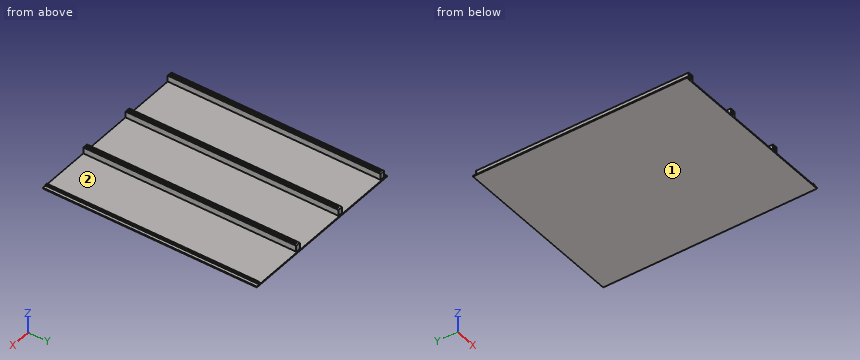
from build123d import *

# Parameters (mm, degrees)
F0_W     = 5.2
F0_H     = 226.71
F1_DEPTH = 2
F3_DEPTH = 4.5
F4_W     = 1.2
F4_H     = 2.1
F5_DEPTH = 25
F6_W     = 185.5
F6_H     = 227.71
F6_W_2   = 2.7
F7_DEPTH = 1
F8_W     = 2
F8_H     = 226.618603
F9_DEPTH = 1
F10_SIZE = 1


with BuildPart() as f1:
    # F0 (on Top) → F1 (new body)
    with BuildSketch(Plane.XY):
        with Locations((2.6, 113.355)):
            Rectangle(F0_W, F0_H)
        with Locations((63.6, 113.355)):
            Rectangle(F0_W, F0_H)
        with Locations((124.6, 113.355)):
            Rectangle(F0_W, F0_H)
    extrude(amount=F1_DEPTH)

    # F2 (on face) → F3 (join)
    with BuildSketch(Plane.XY.offset(2)):
        Polygon((0, 226.71), (0, 0), (2, 0), (2, 224.71), (3.2, 224.71), (3.2, 0), (5.2, 0), (5.2, 226.71), align=None)
        Polygon((61, 226.71), (61, 0), (63, 0), (63, 224.71), (64.2, 224.71), (64.2, 0), (66.2, 0), (66.2, 226.71), align=None)
        Polygon((122, 226.71), (122, 0), (124, 0), (124, 224.71), (125.2, 224.71), (125.2, 0), (127.2, 0), (127.2, 226.71), align=None)
    extrude(amount=F3_DEPTH)

    # F4 (on face) → F5 (cut)
    with BuildSketch(Plane.XY.offset(2)):
        with Locations((2.6, 2.95)):
            Rectangle(F4_W, F4_H)
        with Locations((63.6, 2.95)):
            Rectangle(F4_W, F4_H)
        with Locations((124.6, 2.95)):
            Rectangle(F4_W, F4_H)
    extrude(amount=-F5_DEPTH, mode=Mode.SUBTRACT)

    # F6 (on Top) → F7 (join)
    with BuildSketch(Plane.XY):
        with Locations((92.75, 113.855)):
            Rectangle(F6_W, F6_H)
        with Locations((-1.35, 113.855)):
            Rectangle(F6_W_2, F6_H)
    extrude(amount=-F7_DEPTH)

    # F8 (on face) → F9 (join)
    with BuildSketch(Plane.XY):
        with Locations((181, 113.309301)):
            Rectangle(F8_W, F8_H)
    extrude(amount=F9_DEPTH)

    # F10
    f10_edges = [f1.edges().sort_by_distance(p)[0] for p in [
        (2.6, 0, 2),
        (63.6, 0, 2),
        (124.6, 0, 2),
    ]]
    chamfer(f10_edges, length=F10_SIZE)


solid = f1.part
Read the model definition and answer for the solid it produces. Units are mm, in the model's axes. Face numbers are marked on the shaded views. Round coordinates to 2 decimals unless told otherwise and drop trailing zeros. Write each loop counter-clockwise with the first axis right and the second up, starting at its lowest first coordinate (ties: lowest second). Pieces come first, ordered by that corner, then holes. Notation, with made-up numbers: M -3.5,-26 L 31.5,-26 A20 ccw 31.5,-17 Z; hole C 80.25,-2 d9. An arc over 180 degrees is marked long. Use a Markdown table: item, result.
1) Straight lines are drawn through the part: line 1 along X through (y, z) = (147, 5.75); line 2 along X through (y, z) = (31, 0.25); line 3 along Z through (x, y) = (77.5, 92.5). For each, find the intervals that lie inside material, in ascending order. Write a range as [from, to].
Answers follow:
| item | result |
|---|---|
| line 1 | x = [0, 2], [3.2, 5.2], [61, 63], [64.2, 66.2], [122, 124], [125.2, 127.2] |
| line 2 | x = [0, 5.2], [61, 66.2], [122, 127.2], [180, 182] |
| line 3 | z = [-1, 0] |
2) Flat-ended cylindrical pins translate along their axes: pin 1 (0.8 mm diameter, centred on x = 180.5, z = 0.5, fed in from +Y); pin 2 (2 mm diameter, centred on x = 181, y = 102.5, fed in from +Z); pin 3 (0.6 mm diameter, centred on x = 124.5, y = 69.5, fed in from +Z). Find the tip coordinate at first contact, or state that the pin passes through.
Answers follow:
| item | result |
|---|---|
| pin 1 | stops at y = 226.62 |
| pin 2 | stops at z = 1 |
| pin 3 | stops at z = 2 |
3) The part is cut by section C-C (x = 144). Write down the section's boundary in (y, z), plus the area to 3 significant figures.
Answers follow:
| item | result |
|---|---|
| outline | M 0,-1 L 227.71,-1 L 227.71,0 L 0,0 Z |
| area | 228 mm2 |
4) The part is cut by section A-A (z = 4.75). Write down the section's boundary in (x, y).
Answers follow:
| item | result |
|---|---|
| outline | M 0,0 L 2,0 L 2,224.71 L 3.2,224.71 L 3.2,0 L 5.2,0 L 5.2,226.71 L 0,226.71 Z; M 61,0 L 63,0 L 63,224.71 L 64.2,224.71 L 64.2,0 L 66.2,0 L 66.2,226.71 L 61,226.71 Z; M 122,0 L 124,0 L 124,224.71 L 125.2,224.71 L 125.2,0 L 127.2,0 L 127.2,226.71 L 122,226.71 Z |
5) For a pull along X with two mould halves and no side action, classify the marked faces 1 and 2 as pulls with the +X half, pulls with the -X half, needs draft (parallel to the pull), parting line crosses it, or undercut.
Answers follow:
| item | result |
|---|---|
| face 1 | needs draft |
| face 2 | undercut |
